The model under review builds one solid part; all positions refer to its coordinate system, in mm. Round coordinates to 2 decimals unless told otherwise and drop trailing zeros. Order: outer loops, then holes, each group sorted by start corner. A loop starts at its lowest first (then second) coordinate and runs counter-clockwise, first axis right, second up.
Autodesk Inventor part; units mm, degrees
ref_plane "YZ Plane" through (0, 0, 0) normal (1, 0, 0) x (0, 1, 0)
ref_plane "XZ Plane" through (0, 0, 0) normal (0, 1, 0) x (-1, 0, 0)
ref_plane "XY Plane" through (0, 0, 0) normal (0, 0, 1) x (1, 0, 0)
sketch "Sketch1" plane through (0, 0, 0) normal (0, 1, 0) x (-1, 0, 0)
  line L0 (-90, 95) -> (90, 95)
  line L1 (95, 90) -> (95, -90)
  line L2 (90, -95) -> (-90, -95)
  line L3 (-95, -90) -> (-95, 90)
  line L4 (-37.5033, 38.736) -> (-37.5033, 44.686)
  line L5 (-37.5033, 44.686) -> (14.5465, 44.686)
  line L6 (14.5465, 44.686) -> (14.5465, 38.736)
  line L7 (14.5465, 38.736) -> (-37.5033, 38.736)
  line L8 (-37.4788, -45.2638) -> (-37.4788, -39.3138)
  line L9 (-37.4788, -39.3138) -> (14.5465, -39.3138)
  line L10 (14.5465, -39.3138) -> (14.5465, -45.2638)
  line L11 (14.5465, -45.2638) -> (-37.4788, -45.2638)
  circle A0 centre (41.7215, 73.186) radius 1.2478
  circle A1 centre (73.2215, -0.3141) radius 3.7486
  circle A2 centre (41.7215, -73.8137) radius 1.2732
  circle A3 centre (-42.2782, -73.8137) radius 1.2727
  circle A4 centre (-42.2783, 73.186) radius 1.2728
  circle A5 centre (89.6714, 89.8399) radius 1.5
  circle A6 centre (89.671, -90.1601) radius 1.5
  circle A7 centre (-90.329, -90.1601) radius 1.5
  circle A8 centre (-90.3286, 89.8399) radius 1.5
  arc A9 (90, -95) -> (95, -90) centre (90, -90) ccw
  arc A10 (-95, -90) -> (-90, -95) centre (-90, -90) ccw
  arc A11 (-90, 95) -> (-95, 90) centre (-90, 90) ccw
  arc A12 (95, 90) -> (90, 95) centre (90, 90) ccw
  point P0 (-95, 95)
  point P1 (95, 95)
  point P2 (95, -95)
  point P3 (-95, -95)
  point P4 (0, 0)
  point P5 (0, 0)
  dimension "d4" = 3
  dimension "d0" = 3
  dimension "d1" = 3
  dimension "d2" = 3
  dimension "d3" = 3
  dimension "d6" = 5
  dimension "d7" = 95
  dimension "d8" = 95
  dimension "d9" = 180
  dimension "d10" = 180
  dimension "d11" = 180
  dimension "d12" = 180
  dimension "d13" = 190
  dimension "d14" = 190
  dimension "d15" = 73.5001
  dimension "d16" = 31.5
  dimension "d17" = 95
  dimension "d18" = 95
extrude "Extrusion1" add sketch "Sketch1" along normal blind 3
properties part number "Old case New Board Adapter" material "Glass"
(1) The part is to be moulded in two halves that separate along Z. For faces 1 (the cylindrical face through (94, 1, 93)), 2 (the cylindrical face through (-76.797, 1.479, -1.44)), 3 (the cylindrical face through (93, 1, -94)), say which applies: pulls with the +Z half, pulls with the -Z half, needs draft (parallel to the pull), parting line crosses it, or undercut.
(2) We need section A-A (x = 6). Give the boundary of the cut face in (y, z).
(3) To check wall thickness, follow L1, parallel to Z at x = 42.5, y = 1.9; L2, parallel to Z at x = -9.5, y = 2.45; L3, parallel to Z at x = -73.5, y = 2.35. State the ranges of each line that lie inside material, in increasing order.
(4) Clearance check with a flat-ended pin moving along its axis: P1, Ø1.8, axis at x = -89.67, z = -90.16, coming from the +Y side. State where the tip first meets the part, or that it passes through.
(5) We need section B-B (y = 1.65). Count the separate pieces of the cut face and the enclosed holes in it, and give its area (3 significant figures).
Verdict:
1. face 1: pulls with the +Z half
1. face 2: undercut
1. face 3: pulls with the -Z half
2. outline: (0, -95) - (3, -95) - (3, -45.26) - (0, -45.26) - close; (0, -39.31) - (3, -39.31) - (3, 38.74) - (0, 38.74) - close; (0, 44.69) - (3, 44.69) - (3, 95) - (0, 95) - close
3. L1: z = -95 to -75.07, -72.56 to 71.93, 74.44 to 95
3. L2: z = -95 to -45.26, -39.31 to 38.74, 44.69 to 95
3. L3: z = -95 to -4.05, 3.42 to 95
4. P1: passes through
5. separate pieces: 1
5. enclosed holes: 11
5. area: 35,400 mm2
